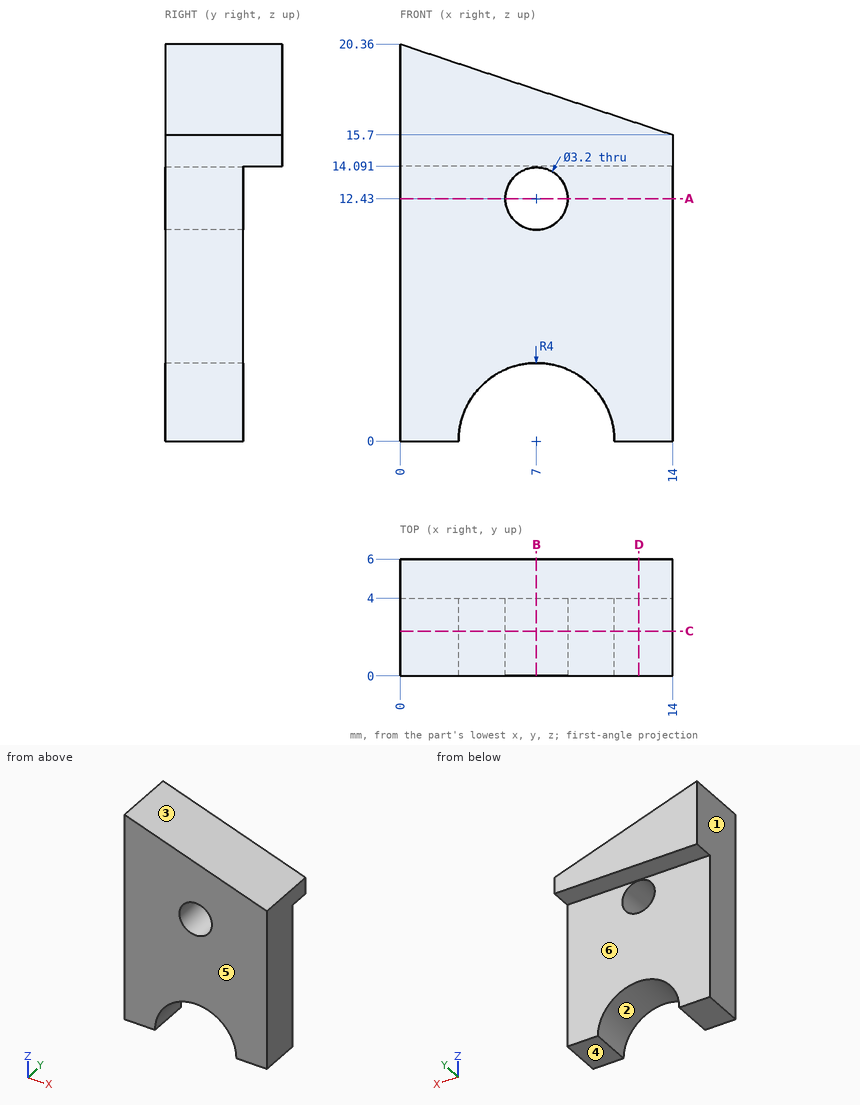
Design review of the part shown in the three views and the two pictorial views. Dimensions are in mm from the part's minimum x, y and z. A direction names the side the tool comes from. Give positions to 0.01 mm unless a question says otherwise; leave off trailing zeros. Write each loop counter-clockwise with the first axis right and the second up, starting at its lowest first coordinate (ties: lowest second). Pieces come first, ordered by that corner, then holes. Notation, with made-up numbers: (88.25, -29) - (98.25, -29) arc R27 cw to (98.25, 4) - close; hole circle Ø2 at (-39, -4.5). An arc over 180 degrees is marked (long way). Return JSON: item names as keys, results as strings. Group by question number.
(1) We need section D-D, the plane x = 12.25. Give the boundary of the cut face in (y, z), then the cut area to 3 significant figures.
(2) We need section C-C, the plane y = 2.3. Give the boundary of the cut face in (x, z), then the cut area to 3 significant figures.
(3) To check wall thickness, follow probe 1 along X at (y, z) = (1.75, 12.43); probe 2 along Y at (x, z) = (3.75, 10); probe 3 along Z at (x, y) = (7, 1.9). State the ranges of each line that lie inside material, in increasing order.
(4) Mouldability with a two-part tool opening along X and no side actions: class the marked faces 1, 2, 3 and 4 as +X half, -X half, draft (parallel to the pull), parting line (faces both ways), or undercut.
(5) We need section B-B, the plane x = 7. Give the boundary of the cut face in (y, z), then the cut area to 3 significant figures.
(6) Machinability: for the marked faces 5 and 6, which of the approach directions +Z, -Z, +X, -X, +Y, -Y give a long, thin tool a straight path to every point of the face, cutting with its end or side? Answer none if there is none.
(7) Insertion check: pin 1 (1 mm diameter, centred on x = 4.5, y = 5, fed in from -Z); pin 2 (1.5 mm diameter, centred on x = 12.5, y = 4.5, fed in from +Z); pin 3 (5 mm diameter, centred on x = 4, z = 3.5, fed in from +Y). Each pin has a flat end and moves straight along its axis. Give the tip position at first contact, or say it passes through.
(8) We need section A-A, the plane z = 12.43. Give the boundary of the cut face in (x, y), then the cut area to 3 significant figures.
Reported:
{
 "1": {"outline": "(0, 0) - (4, 0) - (4, 14.09) - (6, 14.09) - (6, 16.28) - (0, 16.28) - close", "area": "69.5 mm2"},
 "2": {"outline": "(0, 0) - (3, 0) arc R4 cw to (11, 0) - (14, 0) - (14, 15.7) - (0, 20.36) - close; hole circle Ø3.2 at (7, 12.43)", "area": "219 mm2"},
 "3": {"probe 1": "x = 0 to 5.4, 8.6 to 14", "probe 2": "y = 0 to 4", "probe 3": "z = 4 to 10.83, 14.03 to 18.03"},
 "4": {"face 1": "-X half", "face 2": "undercut", "face 3": "+X half", "face 4": "draft"},
 "5": {"outline": "(0, 4) - (4, 4) - (4, 10.83) - (0, 10.83) - close; (0, 14.03) - (4, 14.03) - (4, 14.09) - (6, 14.09) - (6, 18.03) - (0, 18.03) - close", "area": "51.2 mm2"},
 "6": {"face 5": "+Z, -Z, +X, -X, -Y", "face 6": "-Z, +X, -X, +Y"},
 "7": {"pin 1": "stops at z = 14.09", "pin 2": "stops at z = 16.45", "pin 3": "stops at y = 4"},
 "8": {"outline": "(0, 0) - (5.4, 0) - (5.4, 4) - (0, 4) - close; (8.6, 0) - (14, 0) - (14, 4) - (8.6, 4) - close", "area": "43.2 mm2"}
}
